Could you check a few things on this model? Use its own coordinates, in mm. A direction names the side the tool comes from. Round coordinates to 2 decimals unless told otherwise and drop trailing zeros. Write each loop counter-clockwise with the first axis right and the second up, starting at its lowest first coordinate (ties: lowest second). Pieces come first, ordered by that corner, then holes. Notation, with made-up numbers: (-1.5, 21) -> (27.5, 21) arc R23 cw to (27.5, 58) -> close; hole circle Ø10 at (2.5, 2.25). An arc over 180 degrees is marked (long way). One line per question, with ' | ' between items. Start each with the question number.
1. Imagine slicing it at C-C, the plane x = 152. List the corners of the cut face in (y, z) for me, and give its area (3 significant figures).
2. Imagine slicing it at B-B, the plane y = -3. List the corners of the cut face in (x, z) for me, and give its area (3 significant figures).
3. Imagine slicing it at A-A, the plane z = 41. List the corners of the cut face in (x, y) for me, and give its area (3 significant figures).
4. Imagine slicing it at D-D, the plane x = 126.5. List the corners of the cut face in (y, z) for me, and give its area (3 significant figures).
5. For pin 1 Ø1.5 at (y, z) = (-12.5, -1.5) entering from +X; pin 2 Ø8 at (x, y) = (93, -12.5) entering from +Z, each with a flat end and sliding along its axis, tell me the tip position at first contact or that it passes through.
6. If I drill on line 1 along X through (y, z) = (-13, 7); line 2 along X through (y, z) = (-7.5, 45.5); line 3 along Z through (x, y) = (50.5, -14), over which ranges is the centre line in solid material (lowest first)? Write a range as [from, to].
7. For faces 1 (the flat face through (186.14, -12, 21)), 2 (the flat face through (36, -12, 0)), which set-ups out of +Z, -Z, +X, -X, +Y, -Y let a thin tool reach every point of the face, with its end or its side?
8. Thinking about a two-plate mould opening in X: for faces 3 (the flat face through (185.889, -12, -3)), 4 (the flat face through (63, -12, -4.99)), 5 (the flat face through (72.14, -12, 21)), which applies, released by +X, released by -X, zero draft, split by the parting line, or undercut?
from build123d import *

# Parameters (mm, degrees)
F1_DEPTH = 25


# Not quite as in the source:
# - a feature names something its author has since deleted; it is built from what else it names


with BuildPart() as f1:
    # F0 (on Front) → F1 (new body)
    with BuildSketch(Plane.XZ):
        with BuildLine():
            Line((-57.1667980403, 43.3679167181), (-57.1667980403, 0))
            Line((-57.1667980403, 0), (-41.8604705483, 0))
            Line((-41.8604705483, 0), (-41.8604705483, 43.3679167181))
            ThreePointArc((-41.8604705483, 43.3679167181), (-49.5136342943, 48.0061937124), (-57.1667980403, 43.3679167181))
        make_face()
        with BuildLine():
            Line((-0.1667980403, 43.3679167181), (-0.1667980403, 0))
            Line((-0.1667980403, 0), (15.1395294517, 0))
            Line((15.1395294517, 0), (15.1395294517, 43.3679167181))
            ThreePointArc((15.1395294517, 43.3679167181), (7.4863657057, 48.0061937124), (-0.1667980403, 43.3679167181))
        make_face()
        with BuildLine():
            Line((56.8332019597, 43.3679167181), (56.8332019597, 0))
            Line((56.8332019597, 0), (72.1395294517, 0))
            Line((72.1395294517, 0), (72.1395294517, 43.3679167181))
            ThreePointArc((72.1395294517, 43.3679167181), (64.4863657057, 48.0061937124), (56.8332019597, 43.3679167181))
        make_face()
        with BuildLine():
            Line((113.8332019597, 0), (129.1395294517, 0))
            Line((129.1395294517, 0), (129.1395294517, 43.3679167181))
            ThreePointArc((129.1395294517, 43.3679167181), (121.4863657057, 48.0061937124), (113.8332019597, 43.3679167181))
            Line((113.8332019597, 43.3679167181), (113.8332019597, 0))
        make_face()
        with BuildLine():
            Line((170.8332019597, 0), (185.8886182308, 0))
            Line((185.8886182308, 0), (186.1395294517, 0))
            Line((186.1395294517, 0), (186.1395294517, 43.3679167181))
            ThreePointArc((186.1395294517, 43.3679167181), (178.4863657057, 48.0061937124), (170.8332019597, 43.3679167181))
            Line((170.8332019597, 43.3679167181), (170.8332019597, 0))
        make_face()
        Polygon((-41.8604705483, 0), (-57.1667980403, 0), (-57.1667980403, -4.9899439327), (185.8886182308, -4.9899439327), (185.8886182308, 0), (170.8332019597, 0), (162.9481277168, 0), (140.3730809391, 0), (129.1395294517, 0), (113.8332019597, 0), (105.9481277168, 0), (83.3730809391, 0), (72.1395294517, 0), (56.8332019597, 0), (48.9481277168, 0), (15.1395294517, 0), (-0.1667980403, 0), (-8.0518722832, 0), align=None)
    extrude(amount=F1_DEPTH)


solid = f1.part
Geometry results:
1) outline: (-25, -4.99) -> (0, -4.99) -> (0, 0) -> (-25, 0) -> close | area: 125 mm2
2) outline: (-57.17, -4.99) -> (185.89, -4.99) -> (185.89, 0) -> (186.14, 0) -> (186.14, 43.37) arc R8.63 ccw to (170.83, 43.37) -> (170.83, 0) -> (129.14, 0) -> (129.14, 43.37) arc R8.63 ccw to (113.83, 43.37) -> (113.83, 0) -> (72.14, 0) -> (72.14, 43.37) arc R8.63 ccw to (56.83, 43.37) -> (56.83, 0) -> (15.14, 0) -> (15.14, 43.37) arc R8.63 ccw to (-0.17, 43.37) -> (-0.17, 0) -> (-41.86, 0) -> (-41.86, 43.37) arc R8.63 ccw to (-57.17, 43.37) -> close | area: 4,790 mm2
3) outline: (-57.17, -25) -> (-41.86, -25) -> (-41.86, 0) -> (-57.17, 0) -> close; (-0.17, -25) -> (15.14, -25) -> (15.14, 0) -> (-0.17, 0) -> close; (56.83, -25) -> (72.14, -25) -> (72.14, 0) -> (56.83, 0) -> close; (113.83, -25) -> (129.14, -25) -> (129.14, 0) -> (113.83, 0) -> close; (170.83, -25) -> (186.14, -25) -> (186.14, 0) -> (170.83, 0) -> close | area: 1,910 mm2
4) outline: (-25, -4.99) -> (0, -4.99) -> (0, 46.4) -> (-25, 46.4) -> close | area: 1,280 mm2
5) pin 1: stops at x = 185.89 | pin 2: stops at z = 0
6) line 1: x = [-57.17, -41.86], [-0.17, 15.14], [56.83, 72.14], [113.83, 129.14], [170.83, 186.14] | line 2: x = [-55.6, -43.43], [1.4, 13.57], [58.4, 70.57], [115.4, 127.57], [172.4, 184.57] | line 3: z = [-4.99, 0]
7) face 1: +Z, -Z, +X, +Y, -Y | face 2: +Z, +Y, -Y
8) face 3: released by +X | face 4: zero draft | face 5: undercut
